Part model, mm, in its own coordinate system. Face numbers are marked on the shaded views. A direction names the side the tool comes from. Coordinates: 2 decimals unless noted, no trailing zeros. Order: outer loops, then holes, each group sorted by start corner. A loop starts at its lowest first (then second) coordinate and runs counter-clockwise, first axis right, second up.
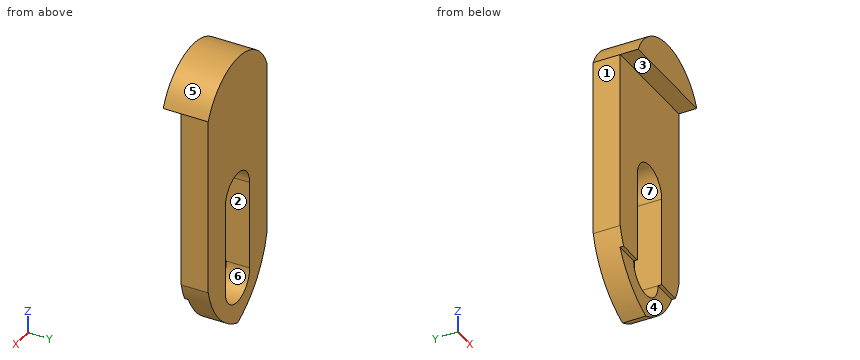
Autodesk Inventor part; units mm, degrees
ref_plane "YZ Plane" through (0, 0, 0) normal (1, 0, 0) x (0, 1, 0)
ref_plane "XZ Plane" through (0, 0, 0) normal (0, 1, 0) x (-1, 0, 0)
ref_plane "XY Plane" through (0, 0, 0) normal (0, 0, 1) x (1, 0, 0)
sketch "Sketch1" plane through (0, 0, 0) normal (0, 1, 0) x (-1, 0, 0)
  line L0 (-3, -8) -> (3, -8)
  line L1 (3, -8) -> (3, 8)
  line L2 (3, 8) -> (-3, 8)
  line L3 (-3, 8) -> (-3, -8)
  line L4 (-3, -8) -> (3, 8) construction
  line L5 (3, -8) -> (-3, 8) construction
  point P0 (0, 0)
  dimension "d0" = 16
  dimension "d1" = 6
extrude "Extrusion1" add sketch "Sketch1" along normal blind 2.5
sketch "Sketch2" plane through (0, 2.5, 0) normal (0, 1, 0) x (1, 0, 0)
  line L0 (0, 5) -> (0, 0) construction
  line L1 (-1.25, 5) -> (-1.25, 0)
  line L2 (1.25, 0) -> (1.25, 5)
  arc A0 (1.25, 5) -> (-1.25, 5) centre (0, 5) ccw
  arc A1 (-1.25, 0) -> (1.25, 0) centre (0, 0) ccw
  line L3 (-3, -8) -> (3, -8)
  line L4 (-3, 8) -> (-3, -8)
  line L5 (-3, -8) -> (3, -8)
  line L6 (3, -8) -> (3, 8)
  line L7 (3, 8) -> (-3, 8)
  point P0 (0, 2.5)
  point P1 (0, 2.5)
  dimension "d4" = 2.5
  dimension "d6" = 8
  dimension "d7" = 6
  dimension "d8" = 3
  dimension "d9" = 5
extrude "Extrusion2" cut sketch "Sketch2" against normal through all contours A0 L2 A1 L1
sketch "Sketch3" plane through (3, 0, 8) normal (1, 0, 0) x (0, 0, -1)
  line L0 (16, 0) -> (0, 0)
  line L1 (16, 0) -> (2, 0)
  line L2 (2, 0) -> (2, 1)
  line L3 (2, 1) -> (16, 1)
  line L4 (16, 1) -> (16, 0)
  line L5 (0, 0) -> (0, 2.5)
  line L6 (0, 2.5) -> (16, 2.5)
  point P0 (8, 0)
  point P1 (2, 0)
  dimension "d12" = 2
  dimension "d13" = 1.5
extrude "Extrusion3" cut sketch "Sketch3" against normal through all
sketch "Sketch4" plane through (0, 2.5, 0) normal (0, 1, 0) x (1, 0, 0)
  line L0 (-3, 8) -> (-3, -8)
  line L1 (3, -8) -> (3, 8)
  arc A0 (-3, -6) -> (3, -6) centre (0, -4.75) ccw
  line L2 (-3, -8) -> (3, -8)
  point P0 (0, 0)
  point P1 (-2, 6)
  point P2 (2, 6)
  point P3 (3, 8)
  point P4 (0, -8)
  point P5 (-2.2361, -8)
  dimension "d17" = 2
extrude "Extrusion4" cut sketch "Sketch4" against normal through all
sketch "Sketch5" plane through (0, 2.5, 0) normal (0, 1, 0) x (1, 0, 0)
  line L0 (3, -6) -> (3, 8)
  line L1 (3, 8) -> (-3, 8)
  line L2 (-3, 8) -> (-3, -6)
  arc A0 (1.25, 5) -> (-1.25, 5) centre (0, 5) ccw
  arc A1 (3, 4) -> (0, 7.5) centre (-1.8689, 2.8624) ccw
  arc A2 (0, 7.5) -> (-3, 4) centre (1.8689, 2.8624) ccw
  point P0 (0, 0)
  point P1 (-3, 6.2041)
  point P2 (0, 6.25)
  point P3 (0, 6.25)
  dimension "d23" = 5
  dimension "d24" = 4
  dimension "d25" = 0.5
extrude "Extrusion5" cut sketch "Sketch5" against normal through all
sketch "Sketch6" plane through (-3, 1, 6) normal (0, -1, 0) x (1, 0, 0)
  line L0 (6.1469, -11) -> (-0.0299, -11)
  line L1 (-0.0299, -11) -> (-0.0299, -13.5)
  line L2 (-0.0299, -13.5) -> (6.1469, -13.5)
  line L3 (6.1469, -13.5) -> (6.1469, -11)
  arc A0 (1.75, -11) -> (4.25, -11) centre (3, -11) ccw
  point P0 (3, -6)
  point P1 (3, -13.5)
  point P2 (1.75, -11)
extrude "Extrusion6" cut sketch "Sketch6" against normal blind 0.2 contours L3 L2 L1 L0 A0
properties part number "Carrier Tab"
Q1. Wall check: line 1 along X through (y, z) = (1.35, -0.75); line 2 along X through (y, z) = (1.4, -4.75); line 3 along Y through (x, z) = (1.75, -0.5). Give the ranges that are in metal, low to high.
Results list:
line 1: x = -3 to -1.25, 1.25 to 3
line 2: x = -2.76 to -1.25, 1.25 to 2.76
line 3: y = 1 to 2.5
Q2. Pin check, flat tip, straight feed: pin 1 Ø1.3 at (x, z) = (-1, -5.5) entering from -Y. Stop position of the tip, or through.
Results list:
pin 1: stops at y = 1
Q3. Cut at D-D on z = -6.5. Write the cut outline in (x, y), and give its area (3 significant figures).
Results list:
outline: (-1.56, 1.2) - (1.56, 1.2) - (1.56, 2.5) - (-1.56, 2.5) - close
area: 4.06 mm2
Q4. Cut at B-B on y = 1.7. Write the cut outline in (x, z), and give its area (3 significant figures).
Results list:
outline: (-3, -4) arc R5 ccw to (0, -7.5) arc R5 ccw to (3, -4) - (3, 6) arc R3.25 ccw to (-3, 6) - close; hole (-1.25, -5) arc R1.25 ccw to (1.25, -5) - (1.25, 0) arc R1.25 ccw to (-1.25, 0) - close
area: 65.3 mm2
Q5. Cut at C-C on y = 0.3. Write the cut outline in (x, z).
Results list:
outline: (-3, 6) - (3, 6) arc R3.25 ccw to start
Q6. Mould opens along X. For the marked faces 4, 5, 6 and 7 say: pulls with the +X half, pulls with the -X half, needs draft (parallel to the pull), parting line crosses it, or undercut.
Results list:
face 4: needs draft
face 5: parting line crosses it
face 6: undercut
face 7: undercut
Q7. Cut at A-A on x = -1. Write the cut outline in (y, z).
Results list:
outline: (0, 6) - (1, 6) - (1, 0.75) - (2.5, 0.75) - (2.5, 7.84) - (0, 7.84) - close; (1.2, -6.96) - (2.5, -6.96) - (2.5, -5.75) - (1.2, -5.75) - close
Q8. Which spindle directions (+Z, -Z, +X, -X, +Y, -Y) get a long thin tool onto all of the face, cutting with end or side? Do the marked faces 1, 2 and 3. Say none if no direction does.
Results list:
face 1: +Z, -Z, -X, +Y, -Y
face 2: +Y, -Y
face 3: -Z, +X, -X, -Y
